The model under review builds one solid part; all positions refer to its coordinate system, in mm. Round coordinates to 2 decimals unless told otherwise and drop trailing zeros. Write each loop counter-clockwise with the first axis right and the second up, starting at its lowest first coordinate (ties: lowest second). Pieces come first, ordered by that corner, then holes.
Item 1: To check wall thickness, follow L1, parallel to Z at x = -18, y = 2.7; L2, parallel to X at y = 2.45, z = 22.5. State the ranges of each line that lie inside material, in increasing order.
Item 2: Clearance check with a flat-ended pin moving along its axis: pin 1 Ø1.5 at (x, y) = (-6.5, 2) entering from +Z. State where the tip first meets the part, or that it passes through.
Item 3: Add section A-A (y = 1.15). Give the boundary of the cut face in (x, z).
Item 4: Add section B-B (x = -3.5). Give the boundary of the cut face in (y, z).
```python
from build123d import *

# Parameters (mm, degrees)
SKETCH1_W           = 42
SKETCH1_H           = 47.5
BOSS_EXTRUDE1_DEPTH = 3
SKETCH2_W           = 20
SKETCH2_H           = 5
CUT_EXTRUDE1_DEPTH  = 5


with BuildPart() as part:
    # Sketch1 → Boss-Extrude1 (new body)
    with BuildSketch(Plane(origin=(0, 0, 0), x_dir=(1, 0, 0), z_dir=(0, 1, 0))):
        Rectangle(SKETCH1_W, SKETCH1_H)
    extrude(amount=BOSS_EXTRUDE1_DEPTH)

    # Sketch2 → Cut-Extrude1 (cut)
    with BuildSketch(Plane(origin=(0, 0, 0), x_dir=(1, 0, 0), z_dir=(0, 1, 0))):
        with Locations((-11, -21.25)):
            Rectangle(SKETCH2_W, SKETCH2_H)
    extrude(amount=CUT_EXTRUDE1_DEPTH, mode=Mode.SUBTRACT)


solid = part.part
```
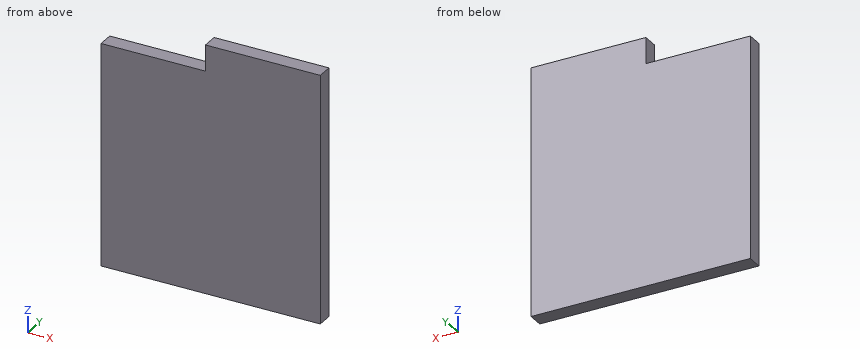
Numbers:
1. L1: z = -23.75 to 18.75
1. L2: x = -1 to 21
2. pin 1: stops at z = 18.75
3. outline: (-21, -23.75) - (21, -23.75) - (21, 23.75) - (-1, 23.75) - (-1, 18.75) - (-21, 18.75) - close
4. outline: (0, -23.75) - (3, -23.75) - (3, 18.75) - (0, 18.75) - close
